```python
from build123d import *

# Parameters (mm, degrees)
F1_DEPTH = 6.35


with BuildPart() as f1:
    # F0 (on Right) → F1 (new body, symmetric)
    with BuildSketch(Plane.YZ):
        with BuildLine():
            ThreePointArc((227.437395, 182.82425), (187.752017, 351.900923), (25.21449, 290.717568))
            Line((25.21449, 290.717568), (-73.912404, 27.874874))
            ThreePointArc((-73.912404, 27.874874), (-37.184675, -69.694705), (64.310285, -45.871988))
            Line((64.310285, -45.871988), (227.437395, 182.82425))
        make_face()
        with BuildLine():
            ThreePointArc((59.140648, -42.184529), (-34.195553, -64.092237), (-67.970892, 25.634128))
            Line((-67.970892, 25.634128), (31.156001, 288.476823))
            ThreePointArc((31.156001, 288.476823), (184.762895, 346.298454), (222.267758, 186.511709))
            Line((222.267758, 186.511709), (59.140648, -42.184529))
        make_face(mode=Mode.SUBTRACT)
    extrude(amount=F1_DEPTH, both=True)


solid = f1.part
```
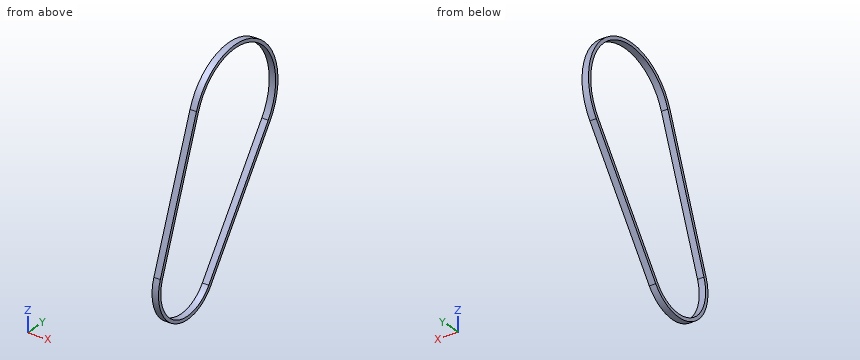
Could you check a few things on this model? Use its own coordinates, in mm. Coordinates: 2 decimals unless noted, no trailing zeros. Order: outer loops, then holes, each group sorted by start corner. A loop starts at its lowest first (then second) coordinate and runs counter-clockwise, first axis right, second up. Notation, with made-up numbers: M 84,55 L 98,55 A20 ccw 98,68 Z; hole C -25.75,-21.5 d7. An arc over 180 degrees is marked long. Use one line per item in the form item = value. Start each with the question number.
1. Suppose I cut it at C-C on z = 238. Write out the boundary of the cut face in (x, y).
2. Suppose I cut it at B-B on x = 0. Write out the boundary of the cut face in (y, z), then the cut area to 3 significant figures.
3. Suppose I cut it at A-A on y = 182. Write out the boundary of the cut face in (x, z), then the cut area to 3 significant figures.
4. For pin 1 (1.5 mm diameter, centred on x = 1, z = 33, fed in from +Y); pin 2 (1.5 mm diameter, centred on x = 3, y = 74.5, fed in from -Z); pin 3 (6 mm diameter, centred on x = 1.5, z = 240, fed in from -Y), each with a flat end and sliding along its axis, tell me the tip position at first contact or that it passes through.
5. Please list where these lines run through material, in increasing order: line 1 (Y direction, x = 0.75, z = 316); line 2 (Y direction, x = 4.5, z = 135); line 3 (Z direction, x = 2, y = 48.5).
Geometry says:
q1.outline = M -6.35,5.33 L 6.35,5.33 L 6.35,12.12 L -6.35,12.12 Z; M -6.35,241.92 L 6.35,241.92 L 6.35,248.3 L -6.35,248.3 Z
q2.outline = M -73.91,27.87 A78.99 ccw 64.31,-45.87 L 227.44,182.82 A115.57 ccw long 25.21,290.72 Z; hole M -67.97,25.63 A72.64 ccw 59.14,-42.18 L 222.27,186.51 A109.22 ccw long 31.16,288.48 Z
q2.area = 7,380 mm^2
q3.outline = M -6.35,119.12 L 6.35,119.12 L 6.35,130.06 L -6.35,130.06 Z; M -6.35,347.72 L 6.35,347.72 L 6.35,354.77 L -6.35,354.77 Z
q3.area = 228 mm^2
q4.pin_1 = 121.1
q4.pin_2 = -32.64
q4.pin_3 = 4.96
q5.line_1 = 38.52 to 46.38, 220.32 to 228.18
q5.line_2 = -33.51 to -26.73, 185.52 to 193.32
q5.line_3 = -62.35 to -54.08, 318.71 to 328.4
